Geometry check sheet. Reference: the model listing, model coordinates, mm. Face numbers are marked on the shaded views. A direction names the side the tool comes from. Give positions to 0.01 mm unless a question says otherwise; leave off trailing zeros. Loops run counter-clockwise (first coordinate to the right, second up) from the corner with the lowest first, then second, coordinate; pieces in that order, holes last.
1. Cross-section at C-C, the plane y = 2.75. Record the cut outline in (x, z).
2. Material ranges on L1, parallel to X at y = 22.5, z = 12.5; L2, parallel to X at y = 8.5, z = -15; L3, parallel to X at y = 20.5, z = -23, recorded low to high.
3. Go/stop test with flat-tipped pins: pin 1 Ø4 at (x, y) = (40, 13) entering from -Z; pin 2 Ø6 at (x, z) = (-77.5, 13) entering from -Y; pin 3 Ø7.5 at (x, z) = (19, 0.5) entering from +Y; pin 4 Ø7.5 at (x, y) = (-112, 17.5) entering from -Z. Record where each tip stops, or that it passes through.
4. Tool access check on the marked faces 4, 5 and 6. Record the directions out of +Z, -Z, +X, -X, +Y, -Y that give a thin tool (end or side, any length) a straight path to the whole face; none if there is none.
5. Release check for a two-part mould opening along X. For the marked faces 1, 2 and 3 record: +X half, -X half, draft (parallel to the pull), parting line (faces both ways), or undercut.
6. Cross-section at D-D, the plane x = -51.5. Record the cut outline in (y, z).
7. Cross-section at A-A, the plane y = 22.5. Record the cut outline in (x, z), plus the area to 3 significant figures.
8. Cross-section at B-B, the plane z = -1. Record the cut outline in (x, y), plus the area to 4 significant figures.
from build123d import *

# Parameters (mm, degrees)
SKETCH2_W           = 200
SKETCH2_H           = 110
BOSS_EXTRUDE2_DEPTH = 15
SKETCH3_W           = 110
SKETCH3_H           = 25
BOSS_EXTRUDE3_DEPTH = 13
CUT_EXTRUDE1_DEPTH  = 200
SKETCH8_W           = 110
SKETCH8_H           = 25
BOSS_EXTRUDE5_DEPTH = 7
SKETCH9_W           = 15
SKETCH9_H           = 32.5
CUT_EXTRUDE2_DEPTH  = 17.5
SKETCH10_W          = 110
SKETCH10_H          = 25
BOSS_EXTRUDE6_DEPTH = 20
SKETCH11_W          = 15
SKETCH11_H          = 32.5
CUT_EXTRUDE3_DEPTH  = 17.5
CUT_EXTRUDE4_DEPTH  = 20
CUT_EXTRUDE5_DEPTH  = 20
CUT_EXTRUDE11_DEPTH = 1
CUT_EXTRUDE12_DEPTH = 1


with BuildPart() as part:
    # Sketch2 → Boss-Extrude2 (new body)
    with BuildSketch(Plane(origin=(0, 0, 0), x_dir=(1, 0, 0), z_dir=(0, 1, 0))):
        Rectangle(SKETCH2_W, SKETCH2_H)
    extrude(amount=BOSS_EXTRUDE2_DEPTH)

    # Sketch3 → Boss-Extrude3 (add)
    with BuildSketch(Plane(origin=(100, 0, 0), x_dir=(0, 0, -1), z_dir=(1, 0, 0))):
        with Locations((0, 12.5)):
            Rectangle(SKETCH3_W, SKETCH3_H)
    extrude(amount=BOSS_EXTRUDE3_DEPTH)

    # Sketch6 → Cut-Extrude1 (cut)
    with BuildSketch(Plane.ZY.offset(100)):
        Polygon((-55, 0), (-7.5, 15), (-55, 15), align=None)
        Polygon((7.5, 15), (55, 0), (55, 15), align=None)
    extrude(amount=-CUT_EXTRUDE1_DEPTH, mode=Mode.SUBTRACT)

    # Sketch8 → Boss-Extrude5 (add)
    with BuildSketch(Plane(origin=(113, 0, 0), x_dir=(0, 0, -1), z_dir=(1, 0, 0))):
        with Locations((0, 12.5)):
            Rectangle(SKETCH8_W, SKETCH8_H)
    extrude(amount=BOSS_EXTRUDE5_DEPTH)

    # Sketch9 → Cut-Extrude2 (cut)
    with BuildSketch(Plane(origin=(0, 25, 0), x_dir=(1, 0, 0), z_dir=(0, 1, 0))):
        with Locations((110, 0)):
            Rectangle(SKETCH9_W, SKETCH9_H)
    extrude(amount=-CUT_EXTRUDE2_DEPTH, mode=Mode.SUBTRACT)

    # Sketch10 → Boss-Extrude6 (add)
    with BuildSketch(Plane.ZY.offset(100)):
        with Locations((0, 12.5)):
            Rectangle(SKETCH10_W, SKETCH10_H)
    extrude(amount=BOSS_EXTRUDE6_DEPTH)

    # Sketch11 → Cut-Extrude3 (cut)
    with BuildSketch(Plane(origin=(0, 25, 0), x_dir=(1, 0, 0), z_dir=(0, 1, 0))):
        with Locations((-110, 0)):
            Rectangle(SKETCH11_W, SKETCH11_H)
    extrude(amount=-CUT_EXTRUDE3_DEPTH, mode=Mode.SUBTRACT)

    # Sketch12 → Cut-Extrude4 (cut)
    with BuildSketch(Plane.ZY.offset(120)):
        Polygon((20, 25), (55, 0), (55, 25), align=None)
        Polygon((-20, 25), (-55, 25), (-55, 0), align=None)
    extrude(amount=-CUT_EXTRUDE4_DEPTH, mode=Mode.SUBTRACT)

    # Sketch13 → Cut-Extrude5 (cut)
    with BuildSketch(Plane(origin=(120, 0, 0), x_dir=(0, 0, -1), z_dir=(1, 0, 0))):
        Polygon((-20, 25), (-55, 25), (-55, 0), align=None)
        Polygon((20, 25), (55, 0), (55, 25), align=None)
    extrude(amount=-CUT_EXTRUDE5_DEPTH, mode=Mode.SUBTRACT)

    # Sketch17 → Cut-Extrude11 (cut)
    with BuildSketch(Plane(origin=(0, 15.793450882, 4.987405542), x_dir=(1, 0, 0), z_dir=(0, 0.953582665, 0.301131368))):
        with BuildLine():
            Line((-15, -2.634899469), (-5, -2.634899469))
            ThreePointArc((-5, -2.634899469), (-50.541779196, -22.5572379), (-100, -27.540973026))
            ThreePointArc((-100, -27.540973026), (-55.742204199, -21.086980727), (-15, -2.634899469))
        make_face()
        with BuildLine():
            Line((5, -2.634899469), (15, -2.634899469))
            ThreePointArc((15, -2.634899469), (55.742204199, -21.086980727), (100, -27.540973026))
            ThreePointArc((100, -27.540973026), (50.541779196, -22.5572379), (5, -2.634899469))
        make_face()
    extrude(amount=-CUT_EXTRUDE11_DEPTH, mode=Mode.SUBTRACT)

    # Sketch18 → Cut-Extrude12 (cut)
    with BuildSketch(Plane(origin=(0, 15.793450882, -4.987405542), x_dir=(1, 0, 0), z_dir=(0, 0.953582665, -0.301131368))):
        with BuildLine():
            Line((15, 2.634899469), (5, 2.634899469))
            ThreePointArc((5, 2.634899469), (50.541779196, 22.5572379), (100, 27.540973026))
            ThreePointArc((100, 27.540973026), (55.742204199, 21.086980727), (15, 2.634899469))
        make_face()
        with BuildLine():
            Line((-5, 2.634899469), (-15, 2.634899469))
            ThreePointArc((-15, 2.634899469), (-55.742204199, 21.086980727), (-100, 27.540973026))
            ThreePointArc((-100, 27.540973026), (-50.541779196, 22.5572379), (-5, 2.634899469))
        make_face()
    extrude(amount=-CUT_EXTRUDE12_DEPTH, mode=Mode.SUBTRACT)


solid = part.part
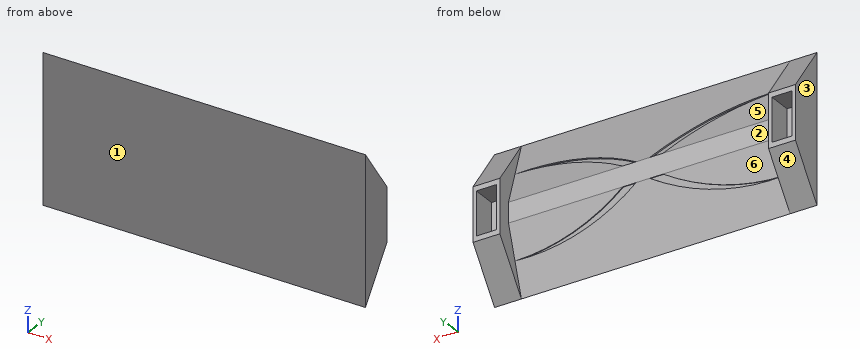
Result:
1. outline: (-120, -51.15) - (-100, -51.15) - (-100, -46.29) - (100, -46.29) - (100, -51.15) - (120, -51.15) - (120, 51.15) - (100, 51.15) - (100, 46.29) - (-100, 46.29) - (-100, 51.15) - (-120, 51.15) - close
2. L1: x = -120 to -117.5, -102.5 to -100, 100 to 102.5, 117.5 to 120
2. L2: x = -120 to -117.5, -102.5 to 102.5, 117.5 to 120
2. L3: x = -120 to -100, 100 to 120
3. pin 1: stops at z = -20.01
3. pin 2: stops at y = 0
3. pin 3: stops at y = 15
3. pin 4: stops at z = -35.75
4. face 4: -Z, +X, -X, +Y
4. face 5: +Z, +Y
4. face 6: -Z, +Y
5. face 1: draft
5. face 2: undercut
5. face 3: -X half
6. outline: (0, -55) - (8.93, -26.73) - (7.97, -26.43) - (8.88, -23.55) - (9.84, -23.85) - (15, -7.5) - (15, 7.5) - (9.84, 23.85) - (8.88, 23.55) - (7.97, 26.43) - (8.93, 26.73) - (0, 55) - close
7. outline: (-120, -23.5) - (-100, -23.5) - (-100, 23.5) - (-120, 23.5) - close; (100, -23.5) - (120, -23.5) - (120, 23.5) - (100, 23.5) - close; hole (-117.5, -16.25) - (-102.5, -16.25) - (-102.5, 16.25) - (-117.5, 16.25) - close; hole (102.5, -16.25) - (117.5, -16.25) - (117.5, 16.25) - (102.5, 16.25) - close
7. area: 905 mm2
8. outline: (-120, 0) - (120, 0) - (120, 25) - (117.5, 25) - (117.5, 7.5) - (102.5, 7.5) - (102.5, 25) - (100, 25) - (100, 15) - (-100, 15) - (-100, 25) - (-102.5, 25) - (-102.5, 7.5) - (-117.5, 7.5) - (-117.5, 25) - (-120, 25) - close
8. area: 3,475 mm2
